from build123d import *

# Parameters (mm, degrees)
CROQUIS1_R                   = 35.5
CROQUIS1_R_2                 = 3.25
SALIENTE_EXTRUIR1_DEPTH      = 5
SALIENTE_EXTRUIR2_DEPTH      = 35
CROQUIS3_R                   = 6
CORTAR_EXTRUIR1_DEPTH        = 65.830018752
CORTAR_EXTRUIR2_REACH        = 42
CROQUIS4_R                   = 1.5
CORTAR_EXTRUIR_L_MINA1_START = 11
CORTAR_EXTRUIR_L_MINA1_DEPTH = 13
CORTAR_EXTRUIR3_REACH        = 83.025
CROQUIS6_R                   = 2
CORTAR_EXTRUIR_L_MINA2_START = 10
CORTAR_EXTRUIR_L_MINA2_DEPTH = 13


with BuildPart() as part:
    # Croquis1 → Saliente-Extruir1 (new body)
    with BuildSketch(Plane.XY):
        Circle(CROQUIS1_R)
        with Locations((17.67766953, 17.67766953)):
            Circle(CROQUIS1_R_2, mode=Mode.SUBTRACT)
        with Locations((17.67766953, -17.67766953)):
            Circle(CROQUIS1_R_2, mode=Mode.SUBTRACT)
        with Locations((-17.67766953, -17.67766953)):
            Circle(CROQUIS1_R_2, mode=Mode.SUBTRACT)
        with Locations((-17.67766953, 17.67766953)):
            Circle(CROQUIS1_R_2, mode=Mode.SUBTRACT)
        Circle(CROQUIS1_R_2, mode=Mode.SUBTRACT)
    extrude(amount=SALIENTE_EXTRUIR1_DEPTH)

    # Croquis2 → Saliente-Extruir2 (add)
    with BuildSketch(Plane.XY.offset(5)):
        with BuildLine():
            ThreePointArc((-29.330018752, -20), (35.5, 0), (-29.330018752, 20))
            Line((-29.330018752, 20), (-29.330018752, -20))
        make_face()
        with BuildLine():
            ThreePointArc((-9.934252718, 17.358301269), (0, 20), (9.934252718, 17.358301268))
            ThreePointArc((9.934252718, 17.358301268), (23.157747084, 23.157747084), (17.358301268, 9.934252718))
            ThreePointArc((17.358301268, 9.934252718), (20, 0), (17.358301268, -9.934252718))
            ThreePointArc((17.358301268, -9.934252718), (23.157747084, -23.157747084), (9.934252718, -17.358301268))
            ThreePointArc((9.934252718, -17.358301268), (0, -20), (-9.934252718, -17.358301268))
            ThreePointArc((-9.934252718, -17.358301268), (-23.157747084, -23.157747084), (-17.358301268, -9.934252718))
            ThreePointArc((-17.358301268, -9.934252718), (-20, 0), (-17.358301269, 9.934252718))
            ThreePointArc((-17.358301269, 9.934252718), (-23.157747084, 23.157747084), (-9.934252718, 17.358301268))
        make_face(mode=Mode.SUBTRACT)
    extrude(amount=SALIENTE_EXTRUIR2_DEPTH)

    # Croquis3 → Cortar-Extruir1 (cut, through all)
    with BuildSketch(Plane.ZY.offset(29.330018752)):
        with Locations((22, 0)):
            Circle(CROQUIS3_R)
    extrude(amount=-CORTAR_EXTRUIR1_DEPTH, mode=Mode.SUBTRACT)

    # Croquis4 → Cortar-Extruir2 (cut, up to next)
    with BuildSketch(Plane.XY.offset(40), mode=Mode.PRIVATE) as cortar_extruir2_sk1:
        with Locations((27.5, 0)):
            Circle(CROQUIS4_R)
    cortar_extruir2_tool1 = extrude(cortar_extruir2_sk1.sketch, amount=-CORTAR_EXTRUIR2_REACH, mode=Mode.PRIVATE) & part.part
    add(cortar_extruir2_tool1.solids().sort_by_distance((27.5, 0, 40))[0], mode=Mode.SUBTRACT)

    # Croquis5 → Cortar-Extruir-Lámina1 (cut)
    with BuildSketch(Plane.XY.offset(5).offset(CORTAR_EXTRUIR_L_MINA1_START)):
        Polygon((-16.202076443, -31.58706569), (-8.717795145, -34.41293431), (-9.4242623, -36.284004634), (-16.908543598, -33.458136015), align=None)
    extrude(amount=CORTAR_EXTRUIR_L_MINA1_DEPTH, mode=Mode.SUBTRACT)

    # Croquis6 → Cortar-Extruir3 (cut, up to next)
    with BuildSketch(Plane(origin=(-12.459935794, -33, 0), x_dir=(0.935535162, -0.353233577, 0), z_dir=(-0.353233577, -0.935535162, 0)), mode=Mode.PRIVATE) as cortar_extruir3_sk1:
        with Locations((0, 22)):
            Circle(CROQUIS6_R)
    cortar_extruir3_tool1 = extrude(cortar_extruir3_sk1.sketch, amount=-CORTAR_EXTRUIR3_REACH, mode=Mode.PRIVATE) & part.part
    add(cortar_extruir3_tool1.solids().sort_by_distance((-12.459936, -33, 22))[0], mode=Mode.SUBTRACT)

    # Croquis7 → Cortar-Extruir-Lámina2 (cut)
    with BuildSketch(Plane.XY.offset(5).offset(CORTAR_EXTRUIR_L_MINA2_START)):
        Polygon((-10.903572782, -17.554038257), (-3.419291484, -20.379906876), (-2.712824329, -18.508836552), (-10.197105627, -15.682967932), align=None)
    extrude(amount=CORTAR_EXTRUIR_L_MINA2_DEPTH, mode=Mode.SUBTRACT)


solid = part.part
Verification items for the finished model (mm, model axes). A direction names the side the tool comes from. Give positions to 0.01 mm unless a question says otherwise; leave off trailing zeros. Order: outer loops, then holes, each group sorted by start corner. A loop starts at its lowest first (then second) coordinate and runs counter-clockwise, first axis right, second up. Notation, with made-up numbers: M -27,-0.5 L 17,-0.5 A14 ccw 17,25.5 Z; hole C -32.75,64.5 d7. An arc over 180 degrees is marked long. Use one line per item in the form item = value. Start each with the question number.
Q1. Section check B-B (x = 0). Enter the section's corners in (y, z), then the cut area to 3 significant figures.
Q2. Access from +Z, -Z, +X, -X, +Y, -Y to the whole of each face (thin tool, end or side, straight path). Record for faces 1 (the cylindrical face through (15.282, -15.481, 2.465)), 2 (the flat face through (-5.997, -19.406, 19.965)), 3 (the cylindrical face through (-23.34, 22.97, 22.26)).
Q3. Scan lines: line 1 along Z through (x, y) = (-8.5, -22.5); line 2 along Y through (x, z) = (-23.5, 22); line 3 along Z through (x, y) = (19.5, 5). Record each from-to range of solid material in increasing order. Write a range as [from, to].
Q4. Mould release check, pull along X, two halves, no side actions. Record for faces 4 (the flat face through (5, 0, 5)), 5 (the flat face through (-29.33, 5, 26)), 6 (the flat face through (24, 0, 40)), 7 (the cylindrical face through (-11.33, -25.52, 20.78)): +X half, -X half, draft (parallel to the pull), parting line (faces both ways), or undercut.
Q5. Section check A-A (y = 0). Enter the section's corners in (x, z).
Q6. Section check D-D (z = 3). Enter the section's corners in (x, y), then the cut area to 3 significant figures.
Q7. Go/stop test with flat-tipped pins: pin 1 Ø3 at (x, y) = (-11, -6) entering from +Z; pin 2 Ø1.5 at (x, z) = (4, 11.5) entering from +Y; pin 3 Ø5 at (x, y) = (-17.68, 17.68) entering from +Z; pin 4 Ø5 at (y, z) = (-10, 14.5) entering from -X. Record where each tip stops, or that it passes through.
Q8. Section check C-C (z = 22). Enter the section's corners in (x, y).
Evaluation:
q1.outline = M -35.5,0 L -3.25,0 L -3.25,5 L -20,5 L -20,40 L -35.5,40 Z; M 3.25,0 L 35.5,0 L 35.5,40 L 20,40 L 20,5 L 3.25,5 Z
q1.area = 1,410 mm2
q2.face_1 = +Z, -Z
q2.face_2 = none
q2.face_3 = +Z
q3.line_1 = [0, 20], [24, 40]
q3.line_2 = [-26.61, -22.79], [-12.56, -6], [6, 12.56], [22.79, 26.61]
q3.line_3 = [0, 18.68], [25.32, 40]
q4.face_4 = undercut
q4.face_5 = -X half
q4.face_6 = draft
q4.face_7 = undercut
q5.outline = M -35.5,0 L -3.25,0 L -3.25,5 L -20,5 L -20,16 L -29.33,16 L -29.33,5 L -35.5,5 Z; M -29.33,28 L -20,28 L -20,40 L -29.33,40 Z; M 3.25,0 L 35.5,0 L 35.5,16 L 20,16 L 20,5 L 3.25,5 Z; M 20,28 L 26,28 L 26,40 L 20,40 Z; M 29,28 L 35.5,28 L 35.5,40 L 29,40 Z
q6.outline = C 0,0 d71; hole C -17.68,-17.68 d6.5; hole C -17.68,17.68 d6.5; hole C 0,0 d6.5; hole C 17.68,-17.68 d6.5; hole C 17.68,17.68 d6.5
q6.area = 3,790 mm2
q7.pin_1 = 5
q7.pin_2 = 35.35
q7.pin_3 = through
q7.pin_4 = -29.33
q8.outline = M -29.33,-20 A35.5 ccw -16.2,-31.59 L -14.33,-32.29 L -9.03,-18.26 L -9.93,-17.92 A7.75 cw long -17.36,-9.93 A20 cw -19.08,-6 L -29.33,-6 Z; M -29.33,6 L -19.08,6 A20 cw -17.36,9.93 A7.75 cw long -9.93,17.36 A20 cw 9.93,17.36 A7.75 cw long 17.36,9.93 A20 cw 19.08,6 L 34.99,6 A35.5 ccw -29.33,20 Z; M -10.59,-33.71 L -8.72,-34.41 A35.5 ccw 34.99,-6 L 19.08,-6 A20 cw 17.36,-9.93 A7.75 cw long 9.93,-17.36 A20 cw -3.18,-19.75 L -3.42,-20.38 L -5.29,-19.67 Z
